For this review, take the finished solid that the model builds, in its own axes (mm). A direction names the side the tool comes from. Coordinates: 2 decimals unless noted, no trailing zeros. Write each loop counter-clockwise with the first axis right and the second up, starting at its lowest first coordinate (ties: lowest second). Pieces come first, ordered by that corner, then holes. Notation, with made-up numbers: M 11,74.5 L 55,74.5 A19 cw 55,86.5 Z; hole C -31.5,35 d3. An arc over 180 degrees is marked long. One line per question, with ' | ' between items.
Autodesk Fusion 360 part; units mm, degrees
sketch "Sketch1" plane through (0, 0, 0) normal (0, 0, 1) x (1, 0, 0) in component "Component"
  line L0 (53.5, -25) -> (-53.5, -25)
  line L1 (-53.5, -25) -> (-53.5, 25)
  line L2 (-53.5, 25) -> (53.5, 25)
  line L3 (53.5, 25) -> (53.5, -25)
  line L4 (53.5, -25) -> (-53.5, 25) construction
  line L5 (-53.5, -25) -> (53.5, 25) construction
  dimension "d1" = 50
  dimension "d2" = 107
extrude "Extrude1" add sketch "Sketch1" along normal blind 12 in component "Component"
sketch "Sketch2" plane through (0, 0, 0) normal (0, 0, -1) x (1, 0, 0) in component "Component"
  line L0 (-53.5, -25) -> (53.5, -25)
  line L1 (53.5, -25) -> (53.5, 25)
  line L2 (53.5, 25) -> (-53.5, 25)
  line L3 (-53.5, 25) -> (-53.5, -25)
  line L4 (55, -27) -> (-55, -27)
  line L5 (-55, -27) -> (-55, 27)
  line L6 (-55, 27) -> (55, 27)
  line L7 (55, 27) -> (55, -27)
  line L8 (55, -27) -> (-55, 27) construction
  line L9 (-55, -27) -> (55, 27) construction
  dimension "d5" = 54
  dimension "d6" = 110
extrude "Extrude2" add sketch "Sketch2" along normal blind 2 contours L0 L1 L2 L3 | L4 L5 L6 L7 in component "Component"
fillet "Fillet1" radius 5 4 edges at (-55, -27, -1) (-55, 27, -1) (55, 27, -1) (55, -27, -1) in component "Component"
fillet "Fillet2" radius 4 4 edges at (53.5, 25, 6) (53.5, -25, 6) (-53.5, -25, 6) (-53.5, 25, 6) in component "Component"
shell "Shell1" thickness 3 removed faces 1 at (-16.5, -8.3333, 12) in component "Component"
chamfer "Chamfer1" distance 2 angle 45 8 edges at (52.3284, -23.8284, 12) (53.5, 0, 12) (52.3284, 23.8284, 12) (0, 25, 12) (-52.3284, 23.8284, 12) (-53.5, 0, 12) (-52.3284, -23.8284, 12) (0, -25, 12) in component "Component"
component "Component" placed x (1, 0, 0) y (0, 1, 0) z (0, 0, 1) at (0, 0, 0)
1) Insertion check: pin 1 Ø3 at (y, z) = (-9, 2.5) entering from +X; pin 2 Ø6 at (x, z) = (-25.5, 3.5) entering from -Y; pin 3 Ø13 at (x, y) = (5, 0) entering from +Z. Each pin has a flat end and moves straight along its axis. Give the tip position at first contact, or say it passes through.
Responses:
pin 1: x = 53.5 | pin 2: y = -25 | pin 3: z = 1
2) To check wall thickness, follow line 1 along Y through (x, z) = (-5, 4.25); line 2 along X through (y, z) = (-12, 5); line 3 along Z through (x, y) = (26, 21.5). State the ranges of each line that lie inside material, in increasing order. Write a range as [from, to].
Responses:
line 1: [-25, -22], [22, 25] | line 2: [-53.5, -50.5], [50.5, 53.5] | line 3: [-2, 1]
3) We need section C-C on y = -16.5. State the section outline as (x, z) points, then the cut area to 3 significant figures.
Responses:
outline: M -55,-2 L 55,-2 L 55,0 L 53.5,0 L 53.5,10 L 51.5,12 L 50.5,12 L 50.5,1 L -50.5,1 L -50.5,12 L -51.5,12 L -53.5,10 L -53.5,0 L -55,0 Z | area: 389 mm^2
4) The part is to be moulded in two halves that separate along X. For faces 6 (the flat face through (-52.5, 0.3, 11)), 7 (the flat face through (50.5, 0, 6)), 8 (the flat face through (53.5, 0, 5)), say which applies: +X half, -X half, draft (parallel to the pull), parting line (faces both ways), or undercut.
Responses:
face 6: -X half | face 7: undercut | face 8: +X half
5) We need section B-B on x = -4.5. State the section outline as (y, z) points, then the cut area to 3 significant figures.
Responses:
outline: M -27,-2 L 27,-2 L 27,0 L 25,0 L 25,10 L 23,12 L 22,12 L 22,1 L -22,1 L -22,12 L -23,12 L -25,10 L -25,0 L -27,0 Z | area: 220 mm^2
6) We need section A-A on z = 4.5. State the section outline as (x, y) points, then the cut area to 3 significant figures.
Responses:
outline: M -53.5,-21 A4 ccw -49.5,-25 L 49.5,-25 A4 ccw 53.5,-21 L 53.5,21 A4 ccw 49.5,25 L -49.5,25 A4 ccw -53.5,21 Z; hole M -50.5,-21 A1 ccw -49.5,-22 L 49.5,-22 A1 ccw 50.5,-21 L 50.5,21 A1 ccw 49.5,22 L -49.5,22 A1 ccw -50.5,21 Z | area: 893 mm^2
7) Machinability: for faces 1 (the flat face through (-1, 22, 6)), 2 (the cylindrical face through (52.359, 23.797, 5.07)), 3 (the flat face through (-1, 25, 5)), 4 (the cylindrical face through (-52.359, -23.797, 5.07)), 5 (the flat face through (-53.5, 0, 5)), which of the approach directions +Z, -Z, +X, -X, +Y, -Y give a long, thin tool a straight path to every point of the face, cutting with its end or side? Answer none if there is none.
Responses:
face 1: +Z | face 2: +Z, +X, +Y | face 3: +Z, +X, -X, +Y | face 4: +Z, -X, -Y | face 5: +Z, -X, +Y, -Y
